Can you work these out from the model? Positions are in its coordinate system, mm. Face numbers are marked on the shaded views. A direction names the side the tool comes from. Give positions to 0.01 mm unless a question says otherwise; leave off trailing zeros. Order: outer loops, then holes, each group sorted by start corner. A loop starts at its lowest first (then second) coordinate and runs counter-clockwise, first axis right, second up. Notation, with made-up numbers: (52, 0.25) - (66, 0.25) arc R9 ccw to (66, 10.25) - close; hole circle Ø10 at (-7, 81). An arc over 180 degrees is marked (long way). Use one line per item in the form item = value. Start each with the question number.
1) Suppose I cut it at B-B, the plane z = -27.5. Write out the boundary of the cut face in (x, y), and give its area (3 significant figures).
2) For pin 1 (5.5 mm diameter, centred on x = 30, z = 71, fed in from +Y) (3 decimals); pin 2 (10 mm diameter, centred on x = 32, z = -55, fed in from -Y); pin 3 (6 mm diameter, centred on x = 26.5, y = 26.5, fed in from +Z); pin 4 (2.5 mm diameter, centred on y = 53, z = 69, fed in from -X), each with a flat end and sliding along its axis, tell me the tip position at first contact or that it passes through.
3) Please list where these lines run through material, in increasing order: probe 1 along Z at (x, y) = (0.5, 50.5); probe 2 along X at (y, z) = (50.5, 62.5).
4) We'd pull the mould along Y, two halves only. Please class the marked faces 1, 2, 3 and 4: released by +Y, released by -Y, zero draft, split by the parting line, or undercut.
5) Suppose I cut it at A-A, the plane x = 6. Write out the boundary of the cut face in (y, z).
6) Which directions (+Z, -Z, +X, -X, +Y, -Y) give clear straight access to the entire face, cutting with the end or side of a thin tool? Please do the marked faces 5 and 6.
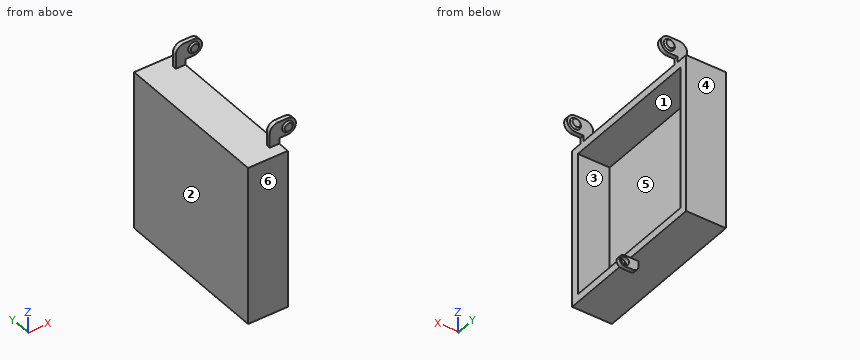
```python
from build123d import *

# Parameters (mm, degrees)
F0_W      = 127
F0_H      = 127
F0_W_2    = 114.3
F0_H_2    = 114.3
F1_DEPTH  = 25.4
F2_W      = 127
F2_H      = 127
F3_DEPTH  = 6.35
F4_W      = 20.8788
F4_H      = 3.302
F5_DEPTH  = 17.78
F6_R      = 6.6294
F8_DEPTH  = 6.35
F9_R      = 6.6294
F10_R     = 4.445
F11_DEPTH = 1.27
F12_R     = 4.445
F13_DEPTH = 1.27
F14_SIZE  = 1.26999
F15_W     = 15.24
F15_H     = 8.89
F16_DEPTH = 1.5875
F17_R     = 4.44499
F18_R     = 3.175
F19_DEPTH = 25.4


# Not quite as in the source:
# - a fillet or chamfer is up to 0.001 mm smaller than in the source, because OpenCascade refuses the exact size
# - a pattern or mirror of a feature is missing from the dataset's text; its kind, count and spacing are read off the source's solid


with BuildPart() as f1:
    # F0 (on Right) → F1 (new body)
    with BuildSketch(Plane.YZ):
        Rectangle(F0_W, F0_H)
        Rectangle(F0_W_2, F0_H_2, mode=Mode.SUBTRACT)
    extrude(amount=F1_DEPTH)

    # F2 (on Right) → F3 (join)
    with BuildSketch(Plane.YZ):
        Rectangle(F2_W, F2_H)
    extrude(amount=-F3_DEPTH)

    # F4 (on face) → F5 (join)
    with BuildSketch(Plane.XY.offset(63.5)):
        with Locations((28.2194, -52.324)):
            Rectangle(F4_W, F4_H)
    f5 = extrude(amount=F5_DEPTH)

    # F5_copies: F5 across plane
    add(f5.mirror(Plane.ZX))

    # F6
    f6_edges = [f1.edges().sort_by_distance(p)[0] for p in [
        (38.6588, -52.324, 81.28),
    ]]
    fillet(f6_edges, radius=F6_R)

    # F7 (on face) → F8 (cut)
    with BuildSketch(Plane.XZ.offset(53.975)):
        with BuildLine():
            ThreePointArc((32.0294, 81.28), (38.6588, 74.6506), (32.0294, 68.0212))
            Line((32.0294, 68.0212), (25.4, 68.0212))
            Line((25.4, 68.0212), (25.4, 63.5))
            Line((25.4, 63.5), (41.4029210806, 57.3826394975))
            Line((41.4029210806, 57.3826394975), (43.7219925225, 87.7940133214))
            Line((43.7219925225, 87.7940133214), (32.0294, 81.28))
        make_face()
    f8 = extrude(amount=-F8_DEPTH, mode=Mode.SUBTRACT)

    # F8_copies: F8 across plane
    add(f8.mirror(Plane.ZX), mode=Mode.SUBTRACT)

    # F9
    f9_edges = [f1.edges().sort_by_distance(p)[0] for p in [
        (17.78, -52.324, 81.28),
        (17.78, 52.324, 81.28),
    ]]
    fillet(f9_edges, radius=F9_R)

    # F10 (on face) → F11 (join)
    with BuildSketch(Plane.XZ.offset(53.975)):
        with Locations((32.0294, 74.6506)):
            Circle(F10_R)
    f11 = extrude(amount=F11_DEPTH)

    # F11_copies: F11 across plane
    add(f11.mirror(Plane.ZX))

    # F12 (on face) → F13 (join)
    with BuildSketch(Plane(origin=(0, -50.673, 0), x_dir=(-1, 0, 0), z_dir=(0, 1, 0))):
        with Locations((-32.0294, 74.6506)):
            Circle(F12_R)
    f13 = extrude(amount=F13_DEPTH)

    # F13_copies: F13 across plane
    add(f13.mirror(Plane.ZX))

    # F14 (size 1.27 in the source; OpenCascade refuses exactly that, so slightly less here)
    f14_edges = [f1.edges().sort_by_distance(p)[0] for p in [
        (27.5844, -55.245, 74.6506),
        (36.4744, -49.403, 74.6506),
        (27.5844, 55.245, 74.6506),
        (36.4744, 49.403, 74.6506),
    ]]
    chamfer(f14_edges, length=F14_SIZE)

    # F15 (on Front) → F16 (join, symmetric)
    with BuildSketch(Plane.XZ):
        with Locations((26.67, -67.945)):
            Rectangle(F15_W, F15_H)
    extrude(amount=F16_DEPTH, both=True)

    # F17 (radius 4.445 in the source; OpenCascade refuses exactly that, so slightly less here)
    f17_edges = [f1.edges().sort_by_distance(p)[0] for p in [
        (34.29, 0, -63.5),
        (34.29, 0, -72.39),
        (19.05, 0, -72.39),
    ]]
    fillet(f17_edges, radius=F17_R)

    # F18 (on face) → F19 (cut)
    with BuildSketch(Plane(origin=(0, 1.5875, 0), x_dir=(-1, 0, 0), z_dir=(0, 1, 0))):
        with Locations((-29.845, -67.945)):
            Circle(F18_R)
    extrude(amount=-F19_DEPTH, mode=Mode.SUBTRACT)


solid = f1.part
```
Result sheet:
q1.outline = (-6.35, -63.5) - (25.4, -63.5) - (25.4, -57.15) - (0, -57.15) - (0, 57.15) - (25.4, 57.15) - (25.4, 63.5) - (-6.35, 63.5) - close
q1.area = 1,130 mm²
q2.pin_1 = 55.245
q2.pin_2 = through
q2.pin_3 = 63.5
q2.pin_4 = 17.78
q3.probe_1 = -63.5 to -57.15, 57.15 to 63.5
q3.probe_2 = -6.35 to 25.4
q4.face_1 = undercut
q4.face_2 = zero draft
q4.face_3 = undercut
q4.face_4 = released by +Y
q5.outline = (-63.5, -63.5) - (63.5, -63.5) - (63.5, 63.5) - (-63.5, 63.5) - close; hole (-57.15, -57.15) - (57.15, -57.15) - (57.15, 57.15) - (-57.15, 57.15) - close
q6.face_5 = +X
q6.face_6 = +Z, -Z, +X, -X, -Y
